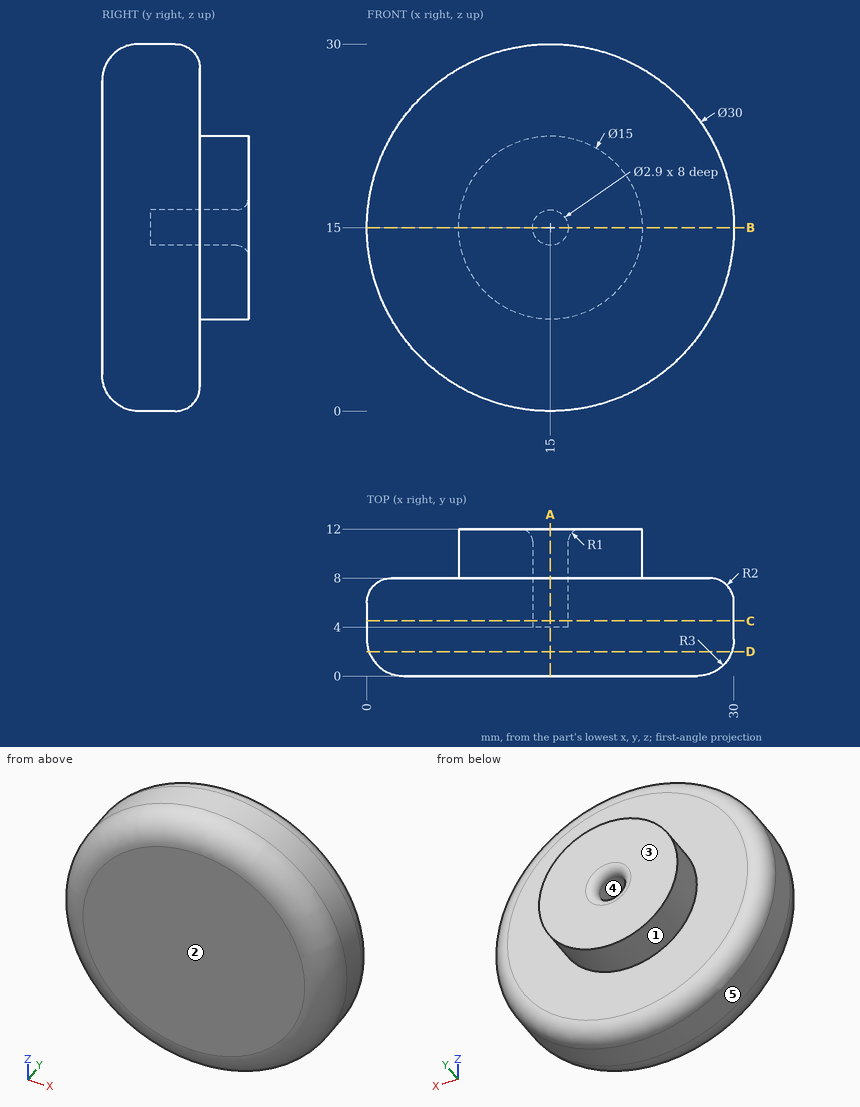
For this review, use the dimensioned drawing (mm, ordinates from the lowest corner) and the shaded views. A direction names the side the tool comes from. Give positions to 0.01 mm unless a question says otherwise; leave off trailing zeros. Loops run counter-clockwise (first coordinate to the right, second up) from the corner with the lowest first, then second, coordinate; pieces in that order, holes last. Notation, with made-up numbers: (-8.5, -32.5) - (36.5, -32.5) arc R26 ccw to (36.5, -3.5) - close; hole circle Ø11 at (51.25, -11.75). An arc over 180 degrees is marked (long way). Write each question's results on one line, items separated by ' | '.
(1) Draft analysis for pull direction Z (two halves, no side actions). For the marked faces 3, 4 and 5, state which applies: +Z half, -Z half, draft (parallel to the pull), parting line (faces both ways), or undercut.
Conclusion:
face 3: draft | face 4: undercut | face 5: parting line
(2) For line 1 along Z through (x, y) = (15, 8.5); line 2 along Z through (x, y) = (15, 6.5); line 3 along Y through (x, z) = (10, 22), list the stretches that pass through material, from the lowest coordinate up.
Conclusion:
line 1: 7.5 to 13.55, 16.45 to 22.5 | line 2: 0.06 to 13.55, 16.45 to 29.94 | line 3: 0 to 8
(3) For pin 1 Ø4 at (y, z) = (2, 17) entering from -X; pin 2 Ø4 at (x, y) = (8.5, 2) entering from -Z; pin 3 Ø6 at (x, z) = (13.5, 3) entering from +Y, all flat-tipped, find the tip position at first contact; note any pin that passes through.
Conclusion:
pin 1: x = 0 | pin 2: z = 0.75 | pin 3: y = 8
(4) Take a section at C-C (y = 4.5). Give the boundary of the cut face in (x, z), then the cut area to 3 significant figures.
Conclusion:
outline: circle Ø30 at (15, 15); hole circle Ø2.9 at (15, 15) | area: 700 mm^2
(5) For the marked faces 1 and 2, list the 3-axis set-ups (+Z, -Z, +X, -X, +Y, -Y) from which the entire face can be reached by the end or side of a thin tool; tool diameter is ignored.
Conclusion:
face 1: +Y | face 2: +Z, -Z, +X, -X, -Y
(6) Take a section at D-D (y = 2). Give the boundary of the cut face in (x, z), then the cut area to 3 significant figures.
Conclusion:
outline: circle Ø29.66 at (15, 15) | area: 691 mm^2
(7) Take a section at A-A (x = 15). Give the boundary of the cut face in (y, z), then the cut area to 3 significant figures.
Conclusion:
outline: (0, 3) arc R3 ccw to (3, 0) - (6, 0) arc R2 ccw to (8, 2) - (8, 7.5) - (12, 7.5) - (12, 12.55) arc R1 ccw to (11, 13.55) - (4, 13.55) - (4, 16.45) - (11, 16.45) arc R1 ccw to (12, 17.45) - (12, 22.5) - (8, 22.5) - (8, 28) arc R2 ccw to (6, 30) - (3, 30) arc R3 ccw to (0, 27) - close | area: 271 mm^2
(8) Take a section at B-B (z = 15). Give the boundary of the cut face in (x, y).
Conclusion:
outline: (0, 3) arc R3 ccw to (3, 0) - (27, 0) arc R3 ccw to (30, 3) - (30, 6) arc R2 ccw to (28, 8) - (22.5, 8) - (22.5, 12) - (17.45, 12) arc R1 ccw to (16.45, 11) - (16.45, 4) - (13.55, 4) - (13.55, 11) arc R1 ccw to (12.55, 12) - (7.5, 12) - (7.5, 8) - (2, 8) arc R2 ccw to (0, 6) - close
